from build123d import *

# Parameters (mm, degrees)
SKETCH1_W           = 100
SKETCH1_H           = 40
SKETCH1_R           = 2
BOSS_EXTRUDE1_DEPTH = 6.35


with BuildPart() as part:
    # Sketch1 → Boss-Extrude1 (new body)
    with BuildSketch(Plane.XY):
        with Locations((50, 20)):
            Rectangle(SKETCH1_W, SKETCH1_H)
        with Locations((80, 20)):
            Circle(SKETCH1_R, mode=Mode.SUBTRACT)
        with BuildLine():
            Line((8, 32), (33, 32))
            ThreePointArc((33, 32), (35, 30), (33, 28))
            Line((33, 28), (8, 28))
            ThreePointArc((8, 28), (6, 30), (8, 32))
        make_face(mode=Mode.SUBTRACT)
        with BuildLine():
            Line((8, 12), (33, 12))
            ThreePointArc((33, 12), (35, 10), (33, 8))
            Line((33, 8), (8, 8))
            ThreePointArc((8, 8), (6, 10), (8, 12))
        make_face(mode=Mode.SUBTRACT)
    extrude(amount=BOSS_EXTRUDE1_DEPTH)


solid = part.part
Design review of the part built by this model. Coordinates are the model's own, in mm. A direction names the side the tool comes from. Round coordinates to 2 decimals unless told otherwise and drop trailing zeros. Write each loop counter-clockwise with the first axis right and the second up, starting at its lowest first coordinate (ties: lowest second). Pieces come first, ordered by that corner, then holes. Notation, with made-up numbers: (-32, 32) - (-3, 32) arc R21 ccw to (-3, 70) - close; hole circle Ø6 at (85, 5). An arc over 180 degrees is marked (long way). Use a Markdown table: item, result. Add a question column.
1. Wall thickness on probe 1 along Y at (x, z) = (80, 2.5); probe 2 along X at (y, z) = (19, 1); probe 3 along X at (y, z) = (9, 1.5): over which ranges is each line inside the solid? List them lowest first.
2. Mouldability with a two-part tool opening along X and no side actions: class faces 1 (the face through (35, 10, 3)), 2 (the face through (49, 40, 3)), 3 (the face through (0, 20, 3)) as +X half, -X half, draft (parallel to the pull), parting line (faces both ways), or undercut.
3. For faces 4 (the face through (6, 10, 3)), 5 (the face through (49, 0, 3)), list the 3-axis set-ups (+Z, -Z, +X, -X, +Y, -Y) from which the entire face can be reached by the end or side of a thin tool; tool diameter is ignored.
4. We need section C-C (y = 10). State the section outline as (x, z) points.
5. We need section A-A (z = 1.5). State the section outline as (x, y) points.
6. Clearance check with a flat-ended pin moving along its axis: pin 1 (10 mm diameter, centred on x = 13, y = 6.5, fed in from -Z). State where the tip first meets the part, or that it passes through.
7. We need section B-B (x = 17.5). State the section outline as (y, z) points.
Output:
| question | item | result |
|---|---|---|
| 1 | probe 1 | y = 0 to 18, 22 to 40 |
| 1 | probe 2 | x = 0 to 78.27, 81.73 to 100 |
| 1 | probe 3 | x = 0 to 6.27, 34.73 to 100 |
| 2 | face 1 | undercut |
| 2 | face 2 | draft |
| 2 | face 3 | -X half |
| 3 | face 4 | +Z, -Z |
| 3 | face 5 | +Z, -Z, +X, -X, -Y |
| 4 | outline | (0, 0) - (6, 0) - (6, 6.35) - (0, 6.35) - close; (35, 0) - (100, 0) - (100, 6.35) - (35, 6.35) - close |
| 5 | outline | (0, 0) - (100, 0) - (100, 40) - (0, 40) - close; hole (8, 8) - (33, 8) arc R2 ccw to (33, 12) - (8, 12) arc R2 ccw to start; hole (8, 28) - (33, 28) arc R2 ccw to (33, 32) - (8, 32) arc R2 ccw to start; hole circle Ø4 at (80, 20) |
| 6 | pin 1 | stops at z = 0 |
| 7 | outline | (0, 0) - (8, 0) - (8, 6.35) - (0, 6.35) - close; (12, 0) - (28, 0) - (28, 6.35) - (12, 6.35) - close; (32, 0) - (40, 0) - (40, 6.35) - (32, 6.35) - close |
